Geometry: final body of the model. Coordinates: model frame, mm. Face numbers are marked on the shaded views. A direction names the side the tool comes from. Coordinates: 2 decimals unless noted, no trailing zeros. Order: outer loops, then holes, each group sorted by start corner. A loop starts at its lowest first (then second) coordinate and runs counter-clockwise, first axis right, second up. Notation, with made-up numbers: (12, 63.25) - (67, 63.25) arc R14 ccw to (67, 81.25) - close; hole circle Ø11 at (-21, 34). An arc over 180 degrees is marked (long way). Use a Markdown table: item, result. Add a question column.
```python
from build123d import *

# Parameters (mm, degrees)
BASEHEAD_DEPTH  = 10
SKE2_R          = 2
HOLE_DEPTH      = 13.701705922
HOLE_DEPTH_BACK = 13.701705922


with BuildPart() as part:
    # BodySke → BaseBody (revolve)
    with BuildSketch(Plane.XY):
        Polygon((0, 0), (0, 8.5), (21.5, 8.5), (22, 8), (45, 8), (47, 6), (50, 6), (50, 0), align=None)
    revolve(axis=Axis((0, 0, 0), (-1, 0, 0)))

    # Ske → BaseHead (add)
    with BuildSketch(Plane.ZY):
        Polygon((0, 12.701705922), (-11, 6.350852961), (-11, -6.350852961), (0, -12.701705922), (11, -6.350852961), (11, 6.350852961), align=None)
    extrude(amount=BASEHEAD_DEPTH)

    # Ske1 → HeadFillet (revolve, cut)
    with BuildSketch(Plane.XY):
        Polygon((-10, 12.701705922), (-9.396657217, 12.701705922), (-10, 10.45), align=None)
    revolve(axis=Axis((0, 0, 0), (-1, 0, 0)), mode=Mode.SUBTRACT)

    # Ske2 → Hole (cut, two sides)
    with BuildSketch(Plane(origin=(0, 0, 0), x_dir=(1, 0, 0), z_dir=(0, 1, 0))) as hole_sk:
        with Locations((41, 0)):
            Circle(SKE2_R)
    extrude(amount=HOLE_DEPTH, mode=Mode.SUBTRACT)
    extrude(hole_sk.sketch, amount=-HOLE_DEPTH_BACK, mode=Mode.SUBTRACT)


solid = part.part
```
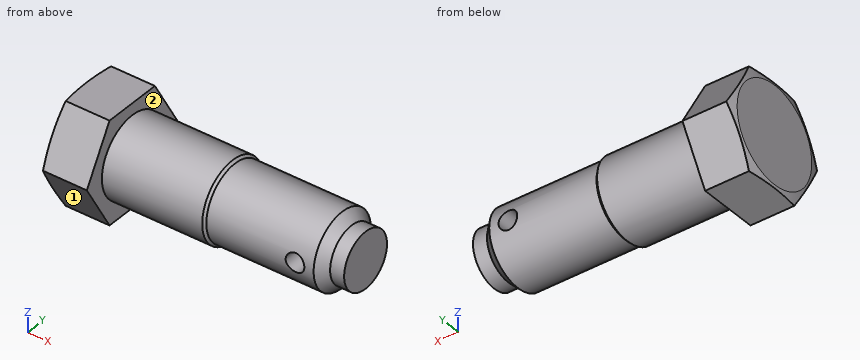
1) Line query: line 1 (X direction, y = 4.25, z = 0); line 2 (Z direction, x = 41, y = -4.5); line 3 (X direction, y = 3, z = 1). Output: solid intervals per line, ascending. Write a range as from..to.
2) Section query A-A (x = 6.5). Return the cut outline in (y, z).
3) Access query for the marked faces 1 and 2. Directions: +Z, -Z, +X, -X, +Y, -Y. A direction counts if a zero-diameter tool reaches every point of the face in a straight line with its end or side. Return the directions, or none.
4) First-contact query: pin 1 (1.5 mm diameter, centred on y = -1, z = 6.5, fed in from +X); pin 2 (1.5 mm diameter, centred on x = 30, z = 3, fed in from -Y); pin 3 (8 mm diameter, centred on x = 29.5, z = -6.5, fed in from -Y); pin 4 (3 mm diameter, centred on x = 41, z = 0, fed in from +Y). Flat tips, straight axial feed; report the tip coordinate or a pass-through.
5) Section query B-B (x = 41). Return the cut outline in (y, z).
From the geometry:
| question | item | result |
|---|---|---|
| 1 | line 1 | x = -10..39, 43..50 |
| 1 | line 2 | z = -6.61..-2, 2..6.61 |
| 1 | line 3 | x = -10..39.27, 42.73..50 |
| 2 | outline | circle Ø17 at (0, 0) |
| 3 | face 1 | -Z, +X, -X, -Y |
| 3 | face 2 | +X |
| 4 | pin 1 | stops at x = 50 |
| 4 | pin 2 | stops at y = -7.68 |
| 4 | pin 3 | stops at y = -7.6 |
| 4 | pin 4 | passes through |
| 5 | outline | (-7.75, -2) arc R8 ccw to (7.75, -2) - close; (-7.75, 2) - (7.75, 2) arc R8 ccw to start |
